Could you check a few things on this model? Use its own coordinates, in mm. Face numbers are marked on the shaded views. A direction names the side the tool comes from. Give positions to 0.01 mm unless a question says otherwise; leave off trailing zeros. Loops run counter-clockwise (first coordinate to the right, second up) from the corner with the lowest first, then second, coordinate; pieces in that order, holes last. Notation, with made-up numbers: (43, 50.5) - (102, 50.5) arc R26 ccw to (102, 88.5) - close; hole circle Ø2 at (62, -20.75). An arc over 180 degrees is marked (long way). One line per item, written item: value. Start each with the question number.
Q1. I'm going to push flat-ended pins straight in: P1, Ø1.1, axis at x = 13, y = 2, coming from the +Z side; P2, Ø1.1, axis at x = 15, y = 1.5, coming from the -Z side; P3, Ø5.5, axis at x = 20.32, z = 0, coming from the +Y side; P4, Ø6, axis at x = -14.5, z = 11, coming from the -Y side. Where does each tip first touch, or does it pass through?
Q2. I want a section at A-A (x = 0). Please give me the cut outline in (y, z) (1 decimal).
Q3. If I drill on line 1 (X direction, y = 2.55, z = 0) (3 decimals); line 2 (Z direction, x = -20.32, y = 1.6); line 3 (Z direction, x = 0, y = 4.5), over which ranges is the centre line in solid material (lowest first)? Write a range as from..to.
Q4. For the marked faces 4 and 5, which set-ups out of +Z, -Z, +X, -X, +Y, -Y let a thin tool reach every point of the face, with its end or its side?
Q5. I want a section at B-B (z = 0). Please give me the cut outline in (x, y) (1 decimal).
Q6. I want a section at D-D (z = -21). Please give me the cut outline in (x, y), then the cut area to 3 significant figures.
Q7. I want a section at C-C (y = 1.5). Please give me the cut outline in (x, z) (3 decimals).
Q8. If we mould it in two halves opening along Z, with no side actions, what happens to the marked faces 1, 2 and 3? For each: released by +Z, released by -Z, zero draft, split by the parting line, or undercut.
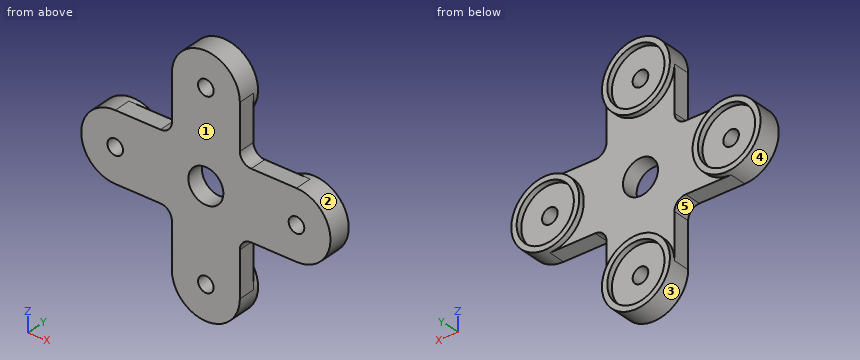
```python
from build123d import *

# Parameters (mm, degrees)
SKETCH1_R                       = 3.925
BOSS_EXTRUDE1_DEPTH             = 3.81
SKETCH1_3_R                     = 6.4135
BOSS_EXTRUDE2_DEPTH             = 5.08
F_5_0_13779528_DIAMETER_HOLE1_D = 3.500000112
CIRPATTERN1_COUNT               = 4
FILLET1_R                       = 2.54


with BuildPart() as part:
    # Sketch1 → Boss-Extrude1 (new body)
    with BuildSketch(Plane(origin=(0, 0, 0), x_dir=(1, 0, 0), z_dir=(0, 1, 0))):
        with BuildLine():
            ThreePointArc((7.62, 20.32), (0, 27.94), (-7.62, 20.32))
            Line((-7.62, 20.32), (-7.62, 6.892838675))
            ThreePointArc((-7.62, 6.892838675), (0, -10.275), (7.62, 6.892838675))
            Line((7.62, 6.892838675), (7.62, 20.32))
        make_face()
        with Locations(Location((0, 0, 0), (0, 0, 90))):
            Circle(SKETCH1_R, mode=Mode.SUBTRACT)
    extrude(amount=BOSS_EXTRUDE1_DEPTH)

    # Sketch1_3 → Boss-Extrude2 (add)
    with BuildSketch(Plane(origin=(0, 0, 0), x_dir=(1, 0, 0), z_dir=(0, 1, 0))):
        with BuildLine():
            ThreePointArc((-7.62, 20.32), (0, 12.7), (7.62, 20.32))
            ThreePointArc((7.62, 20.32), (0, 27.94), (-7.62, 20.32))
        make_face()
        with Locations(Location((0, 20.32, 0), (0, 0, 270))):
            Circle(SKETCH1_3_R, mode=Mode.SUBTRACT)
    extrude(amount=BOSS_EXTRUDE2_DEPTH)

    # 5 _0.13779528_ Diameter Hole1 (through all)
    with Locations(Plane(origin=(0, 3.81, 0), x_dir=(1, 0, 0), z_dir=(0, 1, 0))):
        with Locations((0, 20.32)):
            Hole(F_5_0_13779528_DIAMETER_HOLE1_D / 2)

    # CirPattern1: part ×4 about axis
    cirpattern1_axis = Axis((0, 0, 0), (0, 1, 0))


with BuildPart() as part_1:
    add(part.part)
    for i in range(1, CIRPATTERN1_COUNT):
        add(part.part.rotate(cirpattern1_axis, i * 360 / CIRPATTERN1_COUNT))

    # Fillet1
    fillet1_edges = [part_1.edges().sort_by_distance(p)[0] for p in [
        (7.62, 1.905, -7.62),
        (-7.62, 1.905, 7.62),
        (-7.62, 1.905, -7.62),
        (7.62, 1.905, 7.62),
    ]]
    fillet(fillet1_edges, radius=FILLET1_R)


solid = part_1.part
```
Worked answers:
1. P1: stops at z = 7.62
1. P2: stops at z = -7.62
1. P3: stops at y = 3.81
1. P4: passes through
2. outline: (0, -27.9) - (5.1, -27.9) - (5.1, -26.7) - (3.8, -26.7) - (3.8, -22.1) - (0, -22.1) - close; (0, -18.6) - (3.8, -18.6) - (3.8, -13.9) - (5.1, -13.9) - (5.1, -12.7) - (3.8, -12.7) - (3.8, -3.9) - (0, -3.9) - close; (0, 3.9) - (3.8, 3.9) - (3.8, 12.7) - (5.1, 12.7) - (5.1, 13.9) - (3.8, 13.9) - (3.8, 18.6) - (0, 18.6) - close; (0, 22.1) - (3.8, 22.1) - (3.8, 26.7) - (5.1, 26.7) - (5.1, 27.9) - (0, 27.9) - close
3. line 1: x = -27.94..-22.07, -18.57..-3.925, 3.925..18.57, 22.07..27.94
3. line 2: z = -7.62..-1.75, 1.75..7.62
3. line 3: z = -27.94..-26.73, -13.91..-12.7, 12.7..13.91, 26.73..27.94
4. face 4: +Y
4. face 5: -Z, -X, +Y, -Y
5. outline: (-27.9, 0) - (-22.1, 0) - (-22.1, 3.8) - (-26.7, 3.8) - (-26.7, 5.1) - (-27.9, 5.1) - close; (-18.6, 0) - (-3.9, 0) - (-3.9, 3.8) - (-12.7, 3.8) - (-12.7, 5.1) - (-13.9, 5.1) - (-13.9, 3.8) - (-18.6, 3.8) - close; (3.9, 0) - (18.6, 0) - (18.6, 3.8) - (13.9, 3.8) - (13.9, 5.1) - (12.7, 5.1) - (12.7, 3.8) - (3.9, 3.8) - close; (22.1, 0) - (27.9, 0) - (27.9, 5.1) - (26.7, 5.1) - (26.7, 3.8) - (22.1, 3.8) - close
6. outline: (-7.59, 0) - (-1.61, 0) - (-1.61, 3.81) - (-6.38, 3.81) - (-6.38, 5.08) - (-7.59, 5.08) - close; (1.61, 0) - (7.59, 0) - (7.59, 5.08) - (6.38, 5.08) - (6.38, 3.81) - (1.61, 3.81) - close
6. area: 48.6 mm²
7. outline: (-20.32, -7.62) - (-10.16, -7.62) arc R2.54 cw to (-7.62, -10.16) - (-7.62, -20.32) arc R7.62 ccw to (7.62, -20.32) - (7.62, -10.16) arc R2.54 cw to (10.16, -7.62) - (20.32, -7.62) arc R7.62 ccw to (20.32, 7.62) - (10.16, 7.62) arc R2.54 cw to (7.62, 10.16) - (7.62, 20.32) arc R7.62 ccw to (-7.62, 20.32) - (-7.62, 10.16) arc R2.54 cw to (-10.16, 7.62) - (-20.32, 7.62) arc R7.62 ccw to start; hole circle Ø3.5 at (-20.32, 0); hole circle Ø7.85 at (0, 0); hole circle Ø3.5 at (0, -20.32); hole circle Ø3.5 at (0, 20.32); hole circle Ø3.5 at (20.32, 0)
8. face 1: zero draft
8. face 2: split by the parting line
8. face 3: undercut
